Part print with two shaded views. Sizes in mm from the minimum x, y, z corner. Round coordinates to 2 decimals unless told otherwise and drop trailing zeros. Order: outer loops, then holes, each group sorted by start corner. A loop starts at its lowest first (then second) coordinate and runs counter-clockwise, first axis right, second up. Notation, with made-up numbers: (85.25, 59) -> (100.25, 59) arc R27 ccw to (100.25, 94) -> close; hole circle Ø2 at (88.25, 43). An arc over 180 degrees is marked (long way). Put each result on its own line as item: value. Start each with the question number.
Q1. Flat gauge pins, fed straight in: P1, Ø23, axis at x = 152.4, z = 83.185, coming from the +Y side; P2, Ø1.5, axis at y = 7.5, z = 56, coming from the -X side; P3, Ø5.5, axis at x = 568.5, y = 7.5, coming from the -Z side; P4, Ø5.5, axis at y = 10.5, z = 161.5, coming from the -X side. Where does each tip first touch, or does it go through?
Q2. Cut at A-A, the plane x = 304.8. List the corners of the cut face in (y, z) (3 decimals), and give its area (3 significant figures).
Q3. Probe L1, parallel to X at y = 14, z = 82; L2, parallel to Z at x = 457.2, y = 13.75 (3 decimals); L3, parallel to Z at x = 321, y = 9.75. List the from-to ranges inside material, lowest first.
Q4. Cut at B-B, the plane z = 16.5. List the corners of the cut face in (x, y), and give its area (3 significant figures).
Q5. Cut at C-C, the plane y = 6.5. State how many separate pieces and enclosed holes the cut face has, and give its area (3 significant figures).
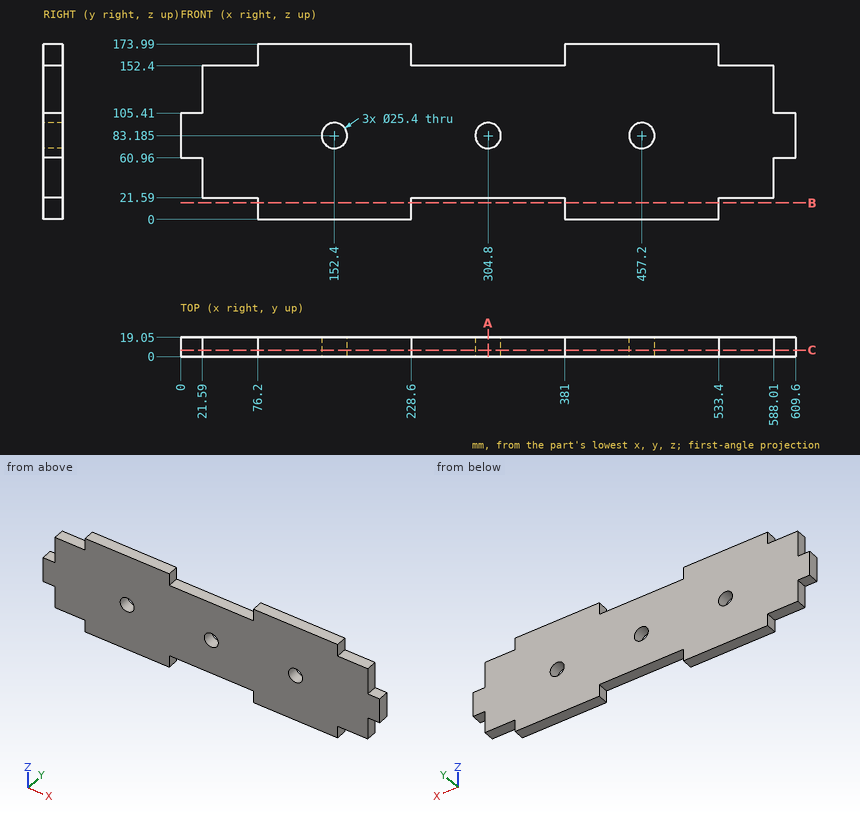
Ans:
1. P1: passes through
1. P2: stops at x = 21.59
1. P3: stops at z = 21.59
1. P4: stops at x = 76.2
2. outline: (0, 21.59) -> (19.05, 21.59) -> (19.05, 70.485) -> (0, 70.485) -> close; (0, 95.885) -> (19.05, 95.885) -> (19.05, 152.4) -> (0, 152.4) -> close
2. area: 2,010 mm^2
3. L1: x = 0 to 139.76, 165.04 to 292.16, 317.44 to 444.56, 469.84 to 609.6
3. L2: z = 0 to 70.485, 95.885 to 173.99
3. L3: z = 21.59 to 152.4
4. outline: (76.2, 0) -> (228.6, 0) -> (228.6, 19.05) -> (76.2, 19.05) -> close; (381, 0) -> (533.4, 0) -> (533.4, 19.05) -> (381, 19.05) -> close
4. area: 5,810 mm^2
5. separate pieces: 1
5. enclosed holes: 3
5. area: 87,700 mm^2
